from build123d import *

# Parameters (mm, degrees)
BRIDA_BASE1_DEPTH                = 2
CROQUIS9_R                       = 1.5
CROQUIS9_R_2                     = 1.25
CROQUIS9_R_3                     = 0.75
CROQUIS9_W                       = 20
CROQUIS9_H                       = 25
CORTAR_EXTRUIR2_DEPTH            = 159.836393815
BRIDA_DE_ARISTA1_STRIP_W         = 9
BRIDA_DE_ARISTA1_STRIP_H         = 2
BRIDA_DE_ARISTA1_STRIP_CUT_DEPTH = 150
BRIDA_DE_ARISTA1_DEPTH           = 150
CROQUIS13_R                      = 1.5
CROQUIS13_W                      = 100
CROQUIS13_H                      = 7
CORTAR_EXTRUIR3_DEPTH            = 10
REDONDEO2_R                      = 5


# Sheet-metal steps are written as plain solids
with BuildPart() as part:
    # Croquis base → Brida base1 (new body)
    with BuildSketch(Plane(origin=(0, 0, 0), x_dir=(1, 0, 0), z_dir=(0, 1, 0))):
        Polygon((-140, 75), (-22.9, 75), (52.1, 56), (140, 56), (140, -56), (52.1, -56), (-22.9, -75), (-140, -75), align=None)
    extrude(amount=-BRIDA_BASE1_DEPTH)

    # Croquis9 → Cortar-Extruir2 (cut, through all)
    with BuildSketch(Plane(origin=(0, 0, 0), x_dir=(1, 0, 0), z_dir=(0, 1, 0))):
        with Locations(Location((85.579206262, -48.986389042, 0), (0, 0, 270))):
            Circle(CROQUIS9_R)
        with Locations(Location((100.179206262, -48.986389042, 0), (0, 0, 270))):
            Circle(CROQUIS9_R)
        with Locations(Location((115.179206262, -48.986389042, 0), (0, 0, 270))):
            Circle(CROQUIS9_R)
        with Locations(Location((135.579206262, -48.986389042, 0), (0, 0, 270))):
            Circle(CROQUIS9_R_2)
        with Locations(Location((-124.420793738, -68.986389042, 0), (0, 0, 270))):
            Circle(CROQUIS9_R)
        with Locations(Location((-34.420793738, -68.986389042, 0), (0, 0, 270))):
            Circle(CROQUIS9_R)
        with Locations(Location((-87.420825, -64, 0), (0, 0, 270))):
            Circle(CROQUIS9_R)
        with Locations(Location((-129.420793738, -41.986389042, 0), (0, 0, 270))):
            Circle(CROQUIS9_R_2)
        with Locations(Location((-43.420793738, -41.986389042, 0), (0, 0, 270))):
            Circle(CROQUIS9_R_2)
        with Locations(Location((60.5792, -43.986389042, 0), (0, 0, 270))):
            Circle(CROQUIS9_R)
        with Locations(Location((135.579206262, -38.986389042, 0), (0, 0, 270))):
            Circle(CROQUIS9_R_2)
        with Locations(Location((134.579206262, -26.986389042, 0), (0, 0, 270))):
            Circle(CROQUIS9_R_2)
        with Locations(Location((-92.420793738, -17.986389042, 0), (0, 0, 270))):
            Circle(CROQUIS9_R_2)
        with Locations(Location((-43.420793738, -17.986389042, 0), (0, 0, 270))):
            Circle(CROQUIS9_R_2)
        with Locations(Location((-21.075793738, -27.986389042, 0), (0, 0, 270))):
            Circle(CROQUIS9_R_2)
        with Locations(Location((27.924206262, -27.986389042, 0), (0, 0, 270))):
            Circle(CROQUIS9_R_2)
        with Locations(Location((64.579206262, -18.986389042, 0), (0, 0, 270))):
            Circle(CROQUIS9_R_2)
        with Locations(Location((114.939206262, -19.846389042, 0), (0, 0, 270))):
            Circle(CROQUIS9_R)
        with Locations(Location((73.219206262, -19.846389042, 0), (0, 0, 270))):
            Circle(CROQUIS9_R)
        with Locations(Location((100.679206262, -8.236389042, 0), (0, 0, 270))):
            Circle(CROQUIS9_R_3)
        with Locations(Location((114.679206262, -8.236389042, 0), (0, 0, 270))):
            Circle(CROQUIS9_R_3)
        with Locations(Location((-124.420793738, 71.013610958, 0), (0, 0, 90))):
            Circle(CROQUIS9_R)
        with Locations(Location((-129.420793738, 44.013610958, 0), (0, 0, 90))):
            Circle(CROQUIS9_R_2)
        with Locations(Location((-87.420825, 66.027221915, 0), (0, 0, 90))):
            Circle(CROQUIS9_R)
        with Locations(Location((-92.420793738, 20.013610958, 0), (0, 0, 90))):
            Circle(CROQUIS9_R_2)
        with Locations(Location((-43.420793738, 20.013610958, 0), (0, 0, 90))):
            Circle(CROQUIS9_R_2)
        with Locations(Location((-43.420793738, 44.013610958, 0), (0, 0, 90))):
            Circle(CROQUIS9_R_2)
        with Locations(Location((-34.420793738, 71.013610958, 0), (0, 0, 90))):
            Circle(CROQUIS9_R)
        with Locations(Location((-21.075793738, 30.013610958, 0), (0, 0, 90))):
            Circle(CROQUIS9_R_2)
        with Locations(Location((115.179206262, 51.013610958, 0), (0, 0, 90))):
            Circle(CROQUIS9_R)
        with Locations(Location((27.924206262, 30.013610958, 0), (0, 0, 90))):
            Circle(CROQUIS9_R_2)
        with Locations(Location((64.579206262, 21.013610958, 0), (0, 0, 90))):
            Circle(CROQUIS9_R_2)
        with Locations(Location((73.219206262, 21.873610958, 0), (0, 0, 90))):
            Circle(CROQUIS9_R)
        with Locations(Location((60.5792, 46.013610958, 0), (0, 0, 90))):
            Circle(CROQUIS9_R)
        with Locations(Location((85.579206262, 51.013610958, 0), (0, 0, 90))):
            Circle(CROQUIS9_R)
        with Locations(Location((100.179206262, 51.013610958, 0), (0, 0, 90))):
            Circle(CROQUIS9_R)
        with Locations(Location((100.679206262, 10.263610958, 0), (0, 0, 90))):
            Circle(CROQUIS9_R_3)
        with Locations(Location((114.679206262, 10.263610958, 0), (0, 0, 90))):
            Circle(CROQUIS9_R_3)
        with Locations(Location((114.939206262, 21.873610958, 0), (0, 0, 90))):
            Circle(CROQUIS9_R)
        with Locations(Location((134.579206262, 29.013610958, 0), (0, 0, 90))):
            Circle(CROQUIS9_R_2)
        with Locations(Location((135.579206262, 41.013610958, 0), (0, 0, 90))):
            Circle(CROQUIS9_R_2)
        with Locations(Location((135.579206262, 51.013610958, 0), (0, 0, 90))):
            Circle(CROQUIS9_R_2)
        with Locations(Location((-129.420793738, 1.013610958, 0), (0, 0, 270))):
            Circle(CROQUIS9_R)
        with Locations((-20.420793738, -48.486389042)):
            Rectangle(CROQUIS9_W, CROQUIS9_H)
        with BuildLine():
            Line((60.579206262, 26.013610958), (60.579206262, -23.986389042))
            ThreePointArc((60.579206262, -23.986389042), (50.579206262, -33.986389042), (40.579206262, -23.986389042))
            Line((40.579206262, -23.986389042), (40.579206262, 26.013610958))
            ThreePointArc((40.579206262, 26.013610958), (50.579206262, 36.013610958), (60.579206262, 26.013610958))
        make_face()
        with Locations((-20.420793738, 50.513610958)):
            Rectangle(CROQUIS9_W, CROQUIS9_H)
    extrude(amount=-CORTAR_EXTRUIR2_DEPTH, mode=Mode.SUBTRACT)

    # Brida de arista1 strip (across the edge) → Brida de arista1 strip cut (cut)
    with BuildSketch(Plane(origin=(-140, -2, 75), x_dir=(1, 0, 0), z_dir=(0, 0, -1))):
        with Locations((-4, -1)):
            Rectangle(BRIDA_DE_ARISTA1_STRIP_W, BRIDA_DE_ARISTA1_STRIP_H)
    extrude(amount=BRIDA_DE_ARISTA1_STRIP_CUT_DEPTH, mode=Mode.SUBTRACT)

    # Brida de arista1 section (across the edge) → Brida de arista1 (add)
    with BuildSketch(Plane(origin=(-140, -2, 75), x_dir=(1, 0, 0), z_dir=(0, 0, -1))):
        with BuildLine():
            Line((-2, 0.5), (-2, 18.4))
            Line((-2, 18.4), (0, 18.4))
            Line((0, 18.4), (0, 0.5))
            ThreePointArc((0, 0.5), (0.146446609, 0.146446609), (0.5, 0))
            Line((0.5, 0), (0.5, -2))
            ThreePointArc((0.5, -2), (-1.267766953, -1.267766953), (-2, 0.5))
        make_face()
    extrude(amount=BRIDA_DE_ARISTA1_DEPTH)

    # Croquis13 → Cortar-Extruir3 (cut)
    with BuildSketch(Plane.ZY.offset(142)):
        with Locations(Location((55, -14.4, 0), (0, 0, 270))):
            Circle(CROQUIS13_R)
        with Locations(Location((-55, -14.4, 0), (0, 0, 270))):
            Circle(CROQUIS13_R)
        with Locations((0, -14.4)):
            Rectangle(CROQUIS13_W, CROQUIS13_H)
    extrude(amount=-CORTAR_EXTRUIR3_DEPTH, mode=Mode.SUBTRACT)

    # Redondeo2
    redondeo2_edges = [part.edges().sort_by_distance(p)[0] for p in [
        (-141, -20.4, 75),
        (-141, -20.4, -75),
    ]]
    fillet(redondeo2_edges, radius=REDONDEO2_R)


solid = part.part
Can you work these out from the model? Positions are in its coordinate system, mm. A direction names the side the tool comes from. Give positions to 0.01 mm unless a question says otherwise; leave off trailing zeros. Loops run counter-clockwise (first coordinate to the right, second up) from the corner with the lowest first, then second, coordinate; pieces in that order, holes last. Notation, with made-up numbers: (-22, 3.25) -> (17, 3.25) arc R24 cw to (17, 14.25) -> close; hole circle Ø11 at (53, 51.5). An arc over 180 degrees is marked (long way). Return JSON: item names as keys, results as strings.
Q1. I want a section at A-A, the plane x = 81.5. List the corners of the cut face in (y, z) for me, then the cut area to 3 significant figures.
Checks:
{"outline": "(-2, -56) -> (0, -56) -> (0, 56) -> (-2, 56) -> close", "area": "224 mm2"}
Q2. I want a section at B-B, the plane y = -6. List the corners of the cut face in (x, z) for me, then the cut area to 3 significant figures.
Checks:
{"outline": "(-142, -75) -> (-140, -75) -> (-140, 75) -> (-142, 75) -> close", "area": "300 mm2"}
Q3. I need wall thicknesses on probe 1 along Y at (x, z) = (-70, -8.5); probe 2 along X at (y, z) = (-7.25, 55); probe 3 along Z at (x, y) = (81, -1.25). Which ranges of each line are inside material? Lowest first, please.
Checks:
{"probe 1": "y = -2 to 0", "probe 2": "x = -142 to -140", "probe 3": "z = -56 to 56"}
Q4. On a 3-axis mill with a long thin cutter (end or side, diameter ignored), from which of +Z, -Z, +X, -X, +Y, -Y can I reach the whole of each face in a straight line? I mean faces 4 (the face through (50.799, -0.986, 33.984)), 5 (the face through (-140.99, -18.9, 73.57)), 6 (the face through (2, -2, -1)). Say none if no direction works.
Checks:
{"face 4": "+Y, -Y", "face 5": "+Z, +X, -X, -Y", "face 6": "+Z, -Z, +X, -Y"}
Q5. We'd pull the mould along X, two halves only. Please class faces 1 (the face through (14.08, -0.99, -65.63)), 2 (the face through (50.36, -0.99, -36.01)), 3 (the face through (2, 0, -1)): released by +X, released by -X, zero draft, split by the parting line, or undercut.
Checks:
{"face 1": "released by +X", "face 2": "undercut", "face 3": "zero draft"}
Q6. For pin 1 Ø2.5 at (x, z) = (100.68, -10.26) entering from +Y; pin 2 Ø10 at (x, y) = (-114, -8) entering from -Z; pin 3 Ø10 at (x, z) = (-20, -21) entering from -Y; pin 4 Ø1 at (y, z) = (-1, -6) entering from -X, each with a flat end and sliding along its axis, tell me the tip position at first contact or that it passes through.
Checks:
{"pin 1": "stops at y = 0", "pin 2": "passes through", "pin 3": "stops at y = -2", "pin 4": "stops at x = -141.79"}
